For this review, use the dimensioned drawing (mm, ordinates from the lowest corner) and the shaded views. Give positions to 0.01 mm unless a question says otherwise; leave off trailing zeros. Loops run counter-clockwise (first coordinate to the right, second up) from the corner with the lowest first, then second, coordinate; pieces in that order, holes last. Notation, with made-up numbers: (10.25, -14.75) - (63.25, -14.75) arc R5 ccw to (63.25, -6.75) - close; hole circle Ø9 at (-0.75, 39.25). An arc over 180 degrees is marked (long way). Write each question's results on one line, items separated by ' | '.
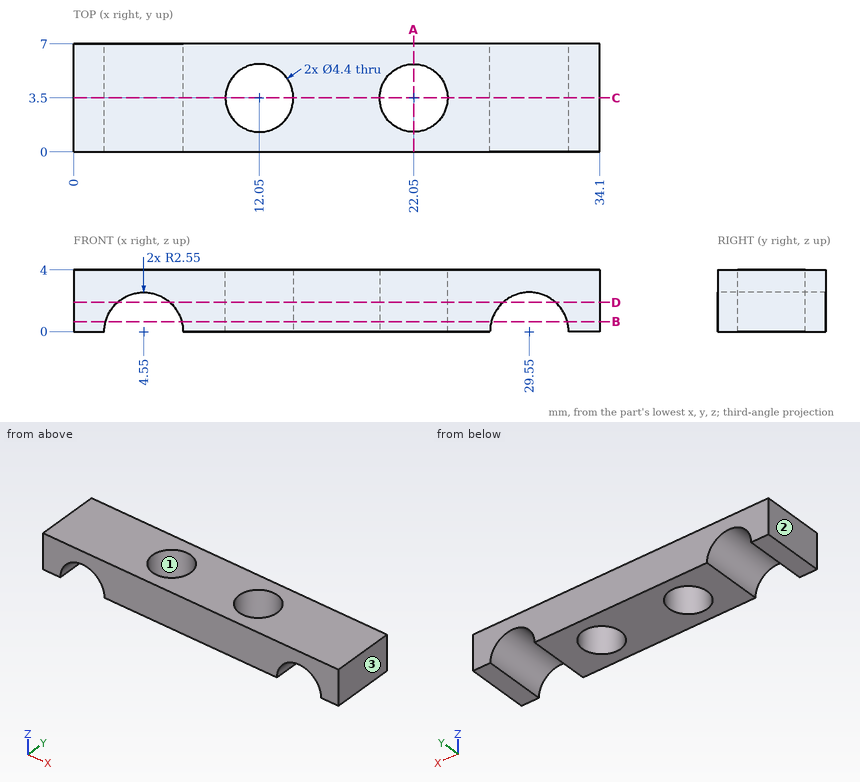
Item 1: We need section D-D on z = 1.9. Give the boundary of the cut face in (x, y), then the cut area to 3 significant figures.
Output values:
outline: (0, 0) - (2.85, 0) - (2.85, 7) - (0, 7) - close; (6.25, 0) - (27.85, 0) - (27.85, 7) - (6.25, 7) - close; (31.25, 0) - (34.1, 0) - (34.1, 7) - (31.25, 7) - close; hole circle Ø4.4 at (12.05, 3.5); hole circle Ø4.4 at (22.05, 3.5) | area: 161 mm²
Item 2: Wall thickness on probe 1 along Y at (x, z) = (12.05, 0.85); probe 2 along X at (y, z) = (5, 0.35); probe 3 along X at (y, z) = (6.5, 1.9): over which ranges is each line inside the solid? List them lowest first.
Output values:
probe 1: y = 0 to 1.3, 5.7 to 7 | probe 2: x = 0 to 2.02, 7.08 to 10.44, 13.66 to 20.44, 23.66 to 27.02, 32.08 to 34.1 | probe 3: x = 0 to 2.85, 6.25 to 27.85, 31.25 to 34.1
Item 3: Clearance check with a flat-ended pin moving along its axis: P1, Ø1.5, axis at x = 20, y = 5, coming from the -Z side. State where the tip first meets the part, or that it passes through.
Output values:
P1: stops at z = 0
Item 4: We need section C-C on y = 3.5. Give the boundary of the cut face in (x, z), then the cut area to 3 significant figures.
Output values:
outline: (0, 0) - (2, 0) arc R2.55 cw to (7.1, 0) - (9.85, 0) - (9.85, 4) - (0, 4) - close; (14.25, 0) - (19.85, 0) - (19.85, 4) - (14.25, 4) - close; (24.25, 0) - (27, 0) arc R2.55 cw to (32.1, 0) - (34.1, 0) - (34.1, 4) - (24.25, 4) - close | area: 80.8 mm²
Item 5: We need section A-A on x = 22.05. Give the boundary of the cut face in (y, z).
Output values:
outline: (0, 0) - (1.3, 0) - (1.3, 4) - (0, 4) - close; (5.7, 0) - (7, 0) - (7, 4) - (5.7, 4) - close
Item 6: We need section B-B on z = 0.65. Give the boundary of the cut face in (x, y), then the cut area to 3 significant figures.
Output values:
outline: (0, 0) - (2.08, 0) - (2.08, 7) - (0, 7) - close; (7.02, 0) - (27.08, 0) - (27.08, 7) - (7.02, 7) - close; (32.02, 0) - (34.1, 0) - (34.1, 7) - (32.02, 7) - close; hole circle Ø4.4 at (12.05, 3.5); hole circle Ø4.4 at (22.05, 3.5) | area: 139 mm²
Item 7: Draft analysis for pull direction X (two halves, no side actions). For the marked faces 1, 2 and 3, state which applies: +X half, -X half, draft (parallel to the pull), parting line (faces both ways), or undercut.
Output values:
face 1: undercut | face 2: -X half | face 3: +X half
